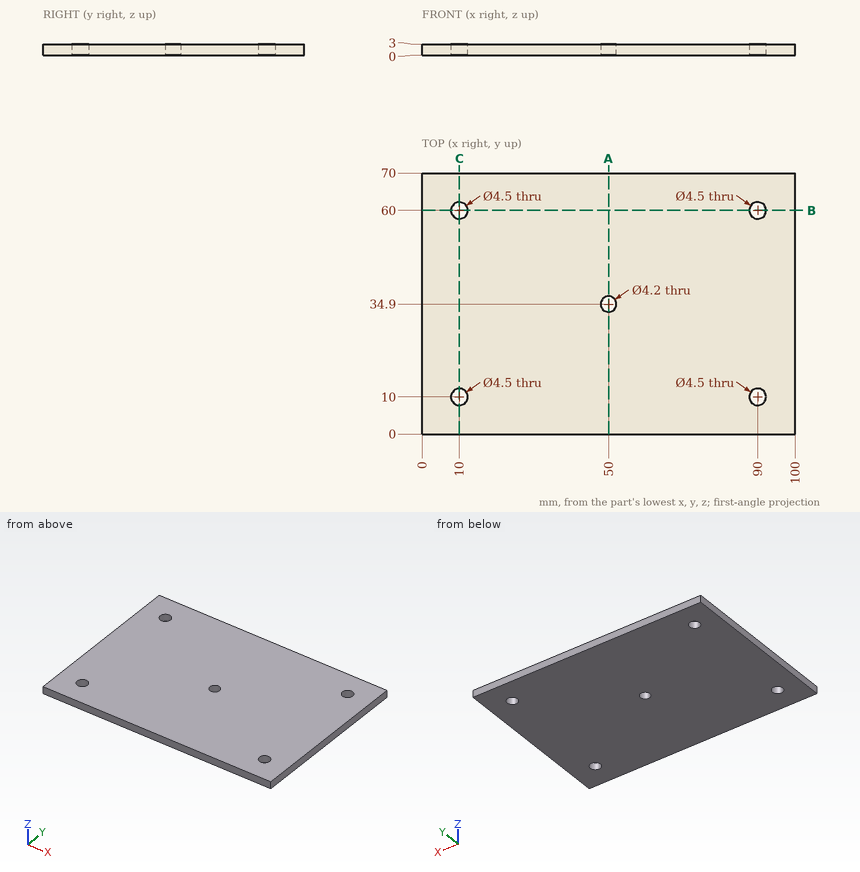
Design review of the part shown in the three views and the two pictorial views. Dimensions are in mm from the part's minimum x, y and z. Coordinates: 2 decimals unless noted, no trailing zeros. Loops run counter-clockwise (first coordinate to the right, second up) from the corner with the lowest first, then second, coordinate; pieces in that order, holes last.
(1) Consider section A-A, the plane x = 50. Give the boundary of the cut face in (y, z), plus the area to 3 significant figures.
Determined:
outline: (0, 0) - (32.8, 0) - (32.8, 3) - (0, 3) - close; (37, 0) - (70, 0) - (70, 3) - (37, 3) - close
area: 197 mm2
(2) Insertion check: P1, Ø4, axis at x = 10, y = 10, coming from the -Z side; P2, Ø3, axis at x = 39, y = 53, coming from the -Z side. Each pin has a flat end and moves straight along its axis. Give the tip position at first contact, or say it passes through.
Determined:
P1: passes through
P2: stops at z = 0
(3) Wall thickness on L1, parallel to Y at x = 88.5, z = 0.75; L2, parallel to X at y = 62, z = 2.15; L3, parallel to Y at x = 8, z = 1.2: over which ranges is each line inside the solid? List them lowest first.
Determined:
L1: y = 0 to 8.32, 11.68 to 58.32, 61.68 to 70
L2: x = 0 to 8.97, 11.03 to 88.97, 91.03 to 100
L3: y = 0 to 8.97, 11.03 to 58.97, 61.03 to 70
(4) Consider section B-B, the plane y = 60. Give the boundary of the cut face in (x, z).
Determined:
outline: (0, 0) - (7.75, 0) - (7.75, 3) - (0, 3) - close; (12.25, 0) - (87.75, 0) - (87.75, 3) - (12.25, 3) - close; (92.25, 0) - (100, 0) - (100, 3) - (92.25, 3) - close
(5) Consider section C-C, the plane x = 10. Give the boundary of the cut face in (y, z).
Determined:
outline: (0, 0) - (7.75, 0) - (7.75, 3) - (0, 3) - close; (12.25, 0) - (57.75, 0) - (57.75, 3) - (12.25, 3) - close; (62.25, 0) - (70, 0) - (70, 3) - (62.25, 3) - close
